Check sheet for the modelled part. Datum: model origin and axes. Units: mm. A direction names the side the tool comes from. Round coordinates to 2 decimals unless told otherwise and drop trailing zeros. Loops run counter-clockwise (first coordinate to the right, second up) from the corner with the lowest first, then second, coordinate; pieces in that order, holes last. Notation, with made-up numbers: M 84.5,64 L 114.5,64 A19 cw 114.5,80 Z; hole C 27,36 d11. An arc over 180 degrees is marked long. Write item = value, one per line. Start each with the question number.
(1) Set-up check for faces 1 (the face through (-28.103, 1.521, -20.789)), 2 (the face through (31, 8, -8)), 3 (the face through (-40.526, 5.465, 11.029)), 4 (the face through (-41, 8, 11)), 5 (the face through (0, 3, 0)): record each of +Z, -Z, +X, -X, +Y, -Y from which the full face is reachable in a straight line by a thin tool's end or side.
(2) Cross-section at B-B on z = -2. Record the boundary of the cut face in (x, y).
(3) Scan lines: L1, parallel to Z at x = 0, y = 38; L2, parallel to Y at x = 14, z = 8.5; L3, parallel to Y at x = 41, z = -15. Record each from-to range of solid material in increasing order. Write a range as from..to.
(4) Cross-section at C-C on x = -15. Record the boundary of the cut face in (y, z).
(5) Go/stop test with flat-tipped pins: P1, Ø8, axis at y = 55.5, z = -7.5, coming from the -X side; P2, Ø8, axis at x = -12, z = 28.5, coming from the +Y side; P3, Ø0.6, axis at x = 32, y = 4.5, coming from the +Z side. Record where each tip stops, or that it passes through.
(6) Mould release check, pull along X, two halves, no side actions. Record for faces 6 (the face through (-29.911, 5.465, 8.143)), 7 (the face through (-42.456, 5.465, 11.554)), 8 (the face through (-5.99, 1.48, 45.61)): pulls with the +X half, pulls with the -X half, needs draft (parallel to the pull), parting line crosses it, or undercut.
(7) Cross-section at A-A on x = 0. Record the boundary of the cut face in (y, z), plus the area to 3 significant figures.
(8) Cross-section at D-D on y = 45. Record the boundary of the cut face in (x, z), plus the area to 3 significant figures.
Autodesk Fusion 360 part; units mm, degrees
sketch "Sketch1" plane through (0, 0, 0) normal (0, 1, 0) x (1, 0, 0)
  circle A0 centre (0, 0) radius 46
  dimension "d1" = 92
extrude "Extrude1" add sketch "Sketch1" along normal blind 3
sketch "Sketch2" plane through (0, 3, 0) normal (0, 1, 0) x (-1, 0, 0)
  circle A0 centre (0, 0) radius 46
  arc A1 (44, 0.0207) -> (38.1051, 22) centre (0, 0) ccw
  arc A2 (-44, 0.0207) -> (-38.1051, -22) centre (0, 0) ccw
  arc A3 (42, 0.0207) -> (36.3731, 21) centre (0, 0) ccw
  arc A4 (-42, 0.0207) -> (-36.3731, -21) centre (0, 0) ccw
  arc A5 (33, 0.0207) -> (28.5788, 16.5) centre (0, 0) ccw
  arc A6 (-33, 0.0207) -> (-28.5788, -16.5) centre (0, 0) ccw
  arc A7 (31, 0.0207) -> (26.8468, 15.5) centre (0, 0) ccw
  arc A8 (-31, 0.0207) -> (-26.8468, -15.5) centre (0, 0) ccw
  line L0 (-26.8468, -15.5) -> (-28.5788, -16.5)
  line L1 (-36.3731, -21) -> (-38.1051, -22)
  line L2 (-31, 0.0207) -> (-33, 0.0207)
  line L3 (-42, 0.0207) -> (-44, 0.0207)
  line L4 (0.0359, 0.0207) -> (0, 0)
  line L5 (44, 0.0207) -> (42, 0.0207)
  line L6 (33, 0.0207) -> (31, 0.0207)
  line L7 (38.1051, 22) -> (36.3731, 21)
  line L8 (28.5788, 16.5) -> (26.8468, 15.5)
  dimension "d8" = 30
  dimension "d9" = 30
  dimension "d23" = 42
  dimension "d24" = 44
  dimension "d25" = 42
  dimension "d26" = 33
  dimension "d27" = 31
  dimension "d28" = 31
  dimension "d29" = 33
extrude "Extrude2" add sketch "Sketch2" along normal blind 5 contours A1 A3 L5 L7 | A2 A4 L1 L3 | A5 A7 L6 L8 | A6 A8 L0 L2
sketch "Sketch3" plane through (0, 3, 0) normal (0, 1, 0) x (-1, 0, 0)
  line L0 (44, 0.0207) -> (42, 0.0207)
  arc A0 (42, 0.0207) -> (36.3731, 21) centre (0, 0) ccw
  line L1 (36.3731, 21) -> (38.1051, 22)
  arc A1 (44, 0.0207) -> (38.1051, 22) centre (0, 0) ccw
  line L2 (-36.3731, -21) -> (-38.1051, -22)
  arc A2 (-44, 0.0207) -> (-38.1051, -22) centre (0, 0) ccw
  line L3 (-44, 0.0207) -> (-42, 0.0207)
  arc A3 (-42, 0.0207) -> (-36.3731, -21) centre (0, 0) ccw
  line L4 (33, 0.0207) -> (31, 0.0207)
  arc A4 (31, 0.0207) -> (26.8468, 15.5) centre (0, 0) ccw
  line L5 (26.8468, 15.5) -> (28.5788, 16.5)
  arc A5 (33, 0.0207) -> (28.5788, 16.5) centre (0, 0) ccw
  line L6 (-26.8468, -15.5) -> (-28.5788, -16.5)
  arc A6 (-33, 0.0207) -> (-28.5788, -16.5) centre (0, 0) ccw
  line L7 (-33, 0.0207) -> (-31, 0.0207)
  arc A7 (-31, 0.0207) -> (-26.8468, -15.5) centre (0, 0) ccw
  circle A8 centre (0, 0) radius 46
  line L8 (-20.4739, -24.5931) -> (-24.3128, -29.2043)
  line L9 (25.5175, -19.3096) -> (30.7614, -22.31)
  arc A9 (-24.3128, -29.2043) -> (30.7614, -22.31) centre (0, 0) ccw
  arc A10 (-20.4739, -24.5931) -> (25.5175, -19.3096) centre (0, 0) ccw
  arc A11 (28, 0.0207) -> (24.2487, 14) centre (0, 0) ccw
  arc A12 (-28, 0.0207) -> (-24.2487, -14) centre (0, 0) ccw
  dimension "d14" = 100
  dimension "d21" = 32
  dimension "d22" = 38
extrude "Extrude3" cut sketch "Sketch3" against normal blind 3 contours L8 L9 A9 A10
sketch "Sketch4" plane through (0, 3, 0) normal (0, 1, 0) x (-1, 0, 0)
  line L0 (25.5175, -19.3096) -> (30.7614, -22.31)
  arc A0 (-24.3128, -29.2043) -> (30.7614, -22.31) centre (0, 0) ccw
  line L1 (-24.3128, -29.2043) -> (-20.4739, -24.5931)
  arc A1 (-20.4739, -24.5931) -> (25.5175, -19.3096) centre (0, 0) ccw
  line L2 (44, 0.0207) -> (42, 0.0207)
  arc A2 (42, 0.0207) -> (36.3731, 21) centre (0, 0) ccw
  line L3 (36.3731, 21) -> (38.1051, 22)
  arc A3 (44, 0.0207) -> (38.1051, 22) centre (0, 0) ccw
  line L4 (-36.3731, -21) -> (-38.1051, -22)
  arc A4 (-44, 0.0207) -> (-38.1051, -22) centre (0, 0) ccw
  line L5 (-44, 0.0207) -> (-42, 0.0207)
  arc A5 (-42, 0.0207) -> (-36.3731, -21) centre (0, 0) ccw
  line L6 (33, 0.0207) -> (31, 0.0207)
  arc A6 (31, 0.0207) -> (26.8468, 15.5) centre (0, 0) ccw
  line L7 (26.8468, 15.5) -> (28.5788, 16.5)
  arc A7 (33, 0.0207) -> (28.5788, 16.5) centre (0, 0) ccw
  line L8 (-26.8468, -15.5) -> (-28.5788, -16.5)
  arc A8 (-33, 0.0207) -> (-28.5788, -16.5) centre (0, 0) ccw
  line L9 (-33, 0.0207) -> (-31, 0.0207)
  arc A9 (-31, 0.0207) -> (-26.8468, -15.5) centre (0, 0) ccw
  circle A10 centre (0, 0) radius 46
  circle A11 centre (0, 0) radius 25
  circle A12 centre (0, 0) radius 23
  dimension "d17" = 50
  dimension "d18" = 46
extrude "Extrude4" add sketch "Sketch4" along normal blind 102 contours A11
sketch "Sketch5" plane through (0, 105, 0) normal (0, 1, 0) x (-1, 0, 0)
  circle A0 centre (0, 0) radius 23
  circle A1 centre (0, 0) radius 25
  circle A2 centre (0, 0) radius 23
extrude "Extrude5" add sketch "Sketch5" against normal blind 2 contours A0 A2
Result:
q1.face_1 = +Y, -Y
q1.face_2 = +Z, -Z, +X, +Y
q1.face_3 = -Z, +Y
q1.face_4 = +Z, -Z, -X, +Y
q1.face_5 = none
q2.outline = M -45.96,0 L 45.96,0 L 45.96,3 L 43.95,3 L 43.95,8 L 41.95,8 L 41.95,3 L 32.94,3 L 32.94,8 L 30.94,8 L 30.94,3 L 24.92,3 L 24.92,105 L -24.92,105 L -24.92,3 L -45.96,3 Z; hole M -22.91,3 L 22.91,3 L 22.91,103 L -22.91,103 Z
q3.L1 = -25..-23, 23..25
q3.L2 = 0..3, 103..105
q3.L3 = 0..8
q4.outline = M 0,-43.49 L 3,-43.49 L 3,-34.91 L 0,-34.91 Z; M 0,-28.27 L 3,-28.27 L 3,-20 L 105,-20 L 105,20 L 3,20 L 3,43.49 L 0,43.49 Z; hole M 3,-17.44 L 103,-17.44 L 103,17.44 L 3,17.44 Z
q5.P1 = -24.75
q5.P2 = 3
q5.P3 = 0.02
q6.face_6 = undercut
q6.face_7 = pulls with the -X half
q6.face_8 = parting line crosses it
q7.outline = M 0,-46 L 3,-46 L 3,-38 L 0,-38 Z; M 0,-32 L 3,-32 L 3,-25 L 105,-25 L 105,25 L 3,25 L 3,46 L 0,46 Z; hole M 3,-23 L 103,-23 L 103,23 L 3,23 Z
q7.area = 758 mm^2
q8.outline = C 0,0 d50; hole C 0,0 d46
q8.area = 302 mm^2
